The listing builds one solid part. Answer for the finished solid, in the listing's coordinates (mm). A direction names the side the tool comes from. Round coordinates to 2 decimals unless told otherwise and drop trailing zeros. Loops run counter-clockwise (first coordinate to the right, second up) from the corner with the lowest first, then second, coordinate; pieces in that order, holes last. Notation, with made-up numbers: (0, 1.5) - (41, 1.5) arc R11 ccw to (41, 21.5) - close; hole circle Ø11 at (-33.5, 1.25). An arc over 180 degrees is marked (long way). One line per item, written item: value.
```python
from build123d import *

# Parameters (mm, degrees)
SKETCH1_R           = 11
BOSS_EXTRUDE1_DEPTH = 60
SKETCH1_3_R         = 6.339
SKETCH1_3_R_2       = 3.302
BOSS_EXTRUDE2_DEPTH = 30
BOSS_EXTRUDE3_DEPTH = 3.175


with BuildPart() as part:
    # Sketch1 → Boss-Extrude1 (new body)
    with BuildSketch(Plane(origin=(0, 0, 0), x_dir=(1, 0, 0), z_dir=(0, 1, 0))):
        with BuildLine():
            ThreePointArc((-5.058299483, 9.767988858), (0, 11), (5.058299483, 9.767988858))
            Line((5.058299483, 9.767988858), (5.058299483, 17.727459811))
            ThreePointArc((5.058299483, 17.727459811), (0, 15.209), (-5.058299483, 17.727459811))
            Line((-5.058299483, 17.727459811), (-5.058299483, 9.767988858))
        make_face()
        with BuildLine():
            ThreePointArc((-9.767988858, -5.058299483), (-11, 0), (-9.767988858, 5.058299483))
            Line((-9.767988858, 5.058299483), (-17.727459811, 5.058299483))
            ThreePointArc((-17.727459811, 5.058299483), (-15.87343723, 2.825289077), (-15.209, 0))
            ThreePointArc((-15.209, 0), (-15.87343723, -2.825289077), (-17.727459811, -5.058299483))
            Line((-17.727459811, -5.058299483), (-9.767988858, -5.058299483))
        make_face()
        Circle(SKETCH1_R)
        with BuildLine():
            ThreePointArc((17.727459811, -5.058299483), (15.209, 0), (17.727459811, 5.058299483))
            Line((17.727459811, 5.058299483), (9.767988858, 5.058299483))
            ThreePointArc((9.767988858, 5.058299483), (10.687559998, 2.603086875), (11, 0))
            ThreePointArc((11, 0), (10.687559998, -2.603086875), (9.767988858, -5.058299483))
            Line((9.767988858, -5.058299483), (17.727459811, -5.058299483))
        make_face()
        with BuildLine():
            Line((5.058299483, -17.727459811), (5.058299483, -9.767988858))
            ThreePointArc((5.058299483, -9.767988858), (0, -11), (-5.058299483, -9.767988858))
            Line((-5.058299483, -9.767988858), (-5.058299483, -17.727459811))
            ThreePointArc((-5.058299483, -17.727459811), (0, -15.209), (5.058299483, -17.727459811))
        make_face()
    extrude(amount=BOSS_EXTRUDE1_DEPTH)

    # Sketch1_3 → Boss-Extrude2 (add)
    with BuildSketch(Plane(origin=(0, 0, 0), x_dir=(1, 0, 0), z_dir=(0, 1, 0))):
        with Locations((21.548, 0)):
            Circle(SKETCH1_3_R)
        with Locations((21.548, 0)):
            Circle(SKETCH1_3_R_2, mode=Mode.SUBTRACT)
        with Locations((0, -21.548)):
            Circle(SKETCH1_3_R)
        with Locations((0, -21.548)):
            Circle(SKETCH1_3_R_2, mode=Mode.SUBTRACT)
        with Locations((-21.548, 0)):
            Circle(SKETCH1_3_R)
        with Locations((-21.548, 0)):
            Circle(SKETCH1_3_R_2, mode=Mode.SUBTRACT)
        with Locations((0, 21.548)):
            Circle(SKETCH1_3_R)
        with Locations((0, 21.548)):
            Circle(SKETCH1_3_R_2, mode=Mode.SUBTRACT)
    extrude(amount=BOSS_EXTRUDE2_DEPTH)

    # Sketch2 → Boss-Extrude3 (add)
    with BuildSketch(Plane(origin=(0, 60, 0), x_dir=(1, 0, 0), z_dir=(0, 1, 0))):
        Polygon((5.773502692, 0), (2.886751346, 5), (-2.886751346, 5), (-5.773502692, 0), (-2.886751346, -5), (2.886751346, -5), align=None)
    extrude(amount=BOSS_EXTRUDE3_DEPTH)


solid = part.part
```
1) A cutting plane is placed at B-B on y = 27.5. Give the vertices of the cut face in (x, z), and give its area (3 significant figures).
Final values:
outline: (-17.73, -5.06) - (-9.77, -5.06) arc R11 ccw to (-5.06, -9.77) - (-5.06, -17.73) arc R6.34 ccw (long way) to (5.06, -17.73) - (5.06, -9.77) arc R11 ccw to (9.77, -5.06) - (17.73, -5.06) arc R6.34 ccw (long way) to (17.73, 5.06) - (9.77, 5.06) arc R11 ccw to (5.06, 9.77) - (5.06, 17.73) arc R6.34 ccw (long way) to (-5.06, 17.73) - (-5.06, 9.77) arc R11 ccw to (-9.77, 5.06) - (-17.73, 5.06) arc R6.34 ccw (long way) to start; hole circle Ø6.6 at (-21.55, 0); hole circle Ø6.6 at (0, -21.55); hole circle Ø6.6 at (0, 21.55); hole circle Ø6.6 at (21.55, 0)
area: 965 mm2
2) Consider L1, parallel to X at y = 21, z = 0; L2, parallel to Z at x = -13, y = 46. Determine where each line is inside the solid, lowest interval first.
Final values:
L1: -27.89 to -24.85, -18.25 to 18.25, 24.85 to 27.89
L2: -5.06 to 5.06
3) A cutting plane is placed at C-C on y = 56.5. Give the vertices of the cut face in (x, z).
Final values:
outline: (-17.73, -5.06) - (-9.77, -5.06) arc R11 ccw to (-5.06, -9.77) - (-5.06, -17.73) arc R6.34 cw to (5.06, -17.73) - (5.06, -9.77) arc R11 ccw to (9.77, -5.06) - (17.73, -5.06) arc R6.34 cw to (17.73, 5.06) - (9.77, 5.06) arc R11 ccw to (5.06, 9.77) - (5.06, 17.73) arc R6.34 cw to (-5.06, 17.73) - (-5.06, 9.77) arc R11 ccw to (-9.77, 5.06) - (-17.73, 5.06) arc R6.34 cw to start
4) A cutting plane is placed at D-D on x = -7.5. Give the vertices of the cut face in (y, z).
Final values:
outline: (0, -8.05) - (60, -8.05) - (60, 8.05) - (0, 8.05) - close
5) For faces 1 (the cylindrical face through (-7.812, 29.58, 7.745)), 2 (the flat face through (4, 60, 4)), 3 (the flat face through (-14, 30, 5.058)), determine the directions among +Z, -Z, +X, -X, +Y, -Y from which every point of the face is accessible in a straight line to the end or side of a thin tool.
Final values:
face 1: +Y, -Y
face 2: +Y
face 3: +Z, +Y, -Y
6) Each of these flat-tipped pins is pushed along its axis until it touches: pin 1 Ø1.5 at (x, y) = (-14.5, 43) entering from +Z; pin 2 Ø12 at (x, z) = (-14.5, 7.5) entering from -Y; pin 3 Ø10 at (x, y) = (7, 25.5) entering from +Z; pin 4 Ø4 at (x, y) = (13, 21.5) entering from -Z. Where does it stop, or does it pass through?
Final values:
pin 1: z = 5.06
pin 2: y = 0
pin 3: z = 27.56
pin 4: z = -5.06
7) For a pull along Z with two mould halves and no side action, classify faces 4 (the cylindrical face through (15.21, 44.79, 0.08)), 5 (the cylindrical face through (-0.08, 44.79, 15.21)), 6 (the flat face through (0, 63.175, 0)) as released by +Z, released by -Z, zero draft, split by the parting line, or undercut.
Final values:
face 4: undercut
face 5: released by +Z
face 6: zero draft
8) A cutting plane is placed at A-A on x = 0. Give the vertices of the cut face in (y, z) (3 decimals), and give its area (3 significant figures).
Final values:
outline: (0, -27.887) - (30, -27.887) - (30, -24.85) - (0, -24.85) - close; (0, -18.246) - (30, -18.246) - (30, -15.209) - (60, -15.209) - (60, -5) - (63.175, -5) - (63.175, 5) - (60, 5) - (60, 15.209) - (30, 15.209) - (30, 18.246) - (0, 18.246) - close; (0, 24.85) - (30, 24.85) - (30, 27.887) - (0, 27.887) - close
area: 2,220 mm2
